Design review of the part built by this model. Coordinates are the model's own, in mm. A direction names the side the tool comes from. Coordinates: 2 decimals unless noted, no trailing zeros. Write each loop counter-clockwise with the first axis right and the second up, starting at its lowest first coordinate (ties: lowest second). Pieces come first, ordered by that corner, then holes. Notation, with made-up numbers: (22.5, -26.5) - (71.5, -26.5) arc R25 cw to (71.5, 1.5) - close; hole circle Ø6 at (40, 72). An arc over 180 degrees is marked (long way). Answer as CSV lines item,"result". Start each with the question number.
Q1. Machinability: for faces 1 (the face through (164.745, 9.658, -105.377)), 2 (the face through (223.617, 25.489, -167.34)), which of the approach directions +Z, -Z, +X, -X, +Y, -Y give a long, thin tool a straight path to every point of the face, cutting with its end or side? Answer none if there is none.
Q2. We need section C-C (y = 7.5). State how many separate pieces and enclosed holes the cut face has, plus the area to 3 significant figures.
Q3. We need section B-B (x = 136.5). Write out the cut boundary in (y, z).
Q4. For line 1 along Z through (x, y) = (47.5, 25.5); line 2 along Z through (x, y) = (46.5, 1.5); line 3 along Z through (x, y) = (91.5, 2), list the stretches that pass through material, from the lowest coordinate up. Write a range as [from, to].
Q5. We need section A-A (z = -25). Write out the cut boundary in (x, y), plus the area to 3 significant figures.
Q6. Mouldability with a two-part tool opening along Z and no side actions: class faces 3 (the face through (105.114, 9.658, -221.512)), 4 (the face through (131.43, 16.61, -271.15)), 5 (the face through (217.3, 9.658, -102.164)), 6 (the face through (269.77, 16.88, 3.14)) as pulls with the +Z half, pulls with the -Z half, needs draft (parallel to the pull), parting line crosses it, or undercut.
Q7. Clearance check with flat-ended pins moving along their axes: pin 1 (10 mm diameter, centred on y = 8, z = -64.5, fed in from -X); pin 2 (13.5 mm diameter, centred on x = 104.98, z = -48.24, fed in from +Y); pin 3 (1 mm diameter, centred on y = 4.5, z = -195, fed in from +X). State where each tip first meets the part, or that it passes through.
from build123d import *

# Parameters (mm, degrees)
SKETCH1_W           = 266.7
SKETCH1_H           = 266.7
BOSS_EXTRUDE1_DEPTH = 31.75
BOSS_EXTRUDE1_DRAFT = -15
SKETCH3_R           = 3.048
CUT_EXTRUDE1_DEPTH  = 31.75
SKETCH4_R           = 7.62
CUT_EXTRUDE2_DEPTH  = 12.7
FILLET1_R           = 5.08
FILLET2_R           = 2.54


with BuildPart() as part:
    # Sketch1 → Boss-Extrude1 (with draft: the straight prism first)
    with BuildSketch(Plane(origin=(0, 0, 0), x_dir=(1, 0, 0), z_dir=(0, 1, 0))):
        with Locations((133.35, 133.35)):
            Rectangle(SKETCH1_W, SKETCH1_H)
    extrude(amount=BOSS_EXTRUDE1_DEPTH)
    # Boss-Extrude1: the draft: its side faces are tilted about the plane it starts from
    boss_extrude1_sides = [part.faces().sort_by_distance(p)[0] for p in [
        (133.35, 15.875, 0),
        (266.7, 15.875, -133.35),
        (133.35, 15.875, -266.7),
        (0, 15.875, -133.35),
    ]]
    draft(boss_extrude1_sides, Plane(origin=(0, 0, 0), x_dir=(1, 0, 0), z_dir=(0, 1, 0)), BOSS_EXTRUDE1_DRAFT)

    # Sketch3 → Cut-Extrude1 (cut)
    with BuildSketch(Plane(origin=(0, 31.75, 0), x_dir=(1, 0, 0), z_dir=(0, 1, 0))):
        with Locations(Location((48.23621314, 48.23621314, 0), (0, 0, 270))):
            Circle(SKETCH3_R)
        with Locations(Location((104.97981314, 48.23621314, 0), (0, 0, 270))):
            Circle(SKETCH3_R)
        with Locations(Location((161.72341314, 48.23621314, 0), (0, 0, 270))):
            Circle(SKETCH3_R)
        with Locations(Location((218.46701314, 48.23621314, 0), (0, 0, 270))):
            Circle(SKETCH3_R)
        with Locations(Location((104.97981314, 104.97981314, 0), (0, 0, 270))):
            Circle(SKETCH3_R)
        with Locations(Location((161.72341314, 104.97981314, 0), (0, 0, 270))):
            Circle(SKETCH3_R)
        with Locations(Location((218.46701314, 104.97981314, 0), (0, 0, 270))):
            Circle(SKETCH3_R)
        with Locations(Location((104.97981314, 161.72341314, 0), (0, 0, 270))):
            Circle(SKETCH3_R)
        with Locations(Location((161.72341314, 161.72341314, 0), (0, 0, 270))):
            Circle(SKETCH3_R)
        with Locations(Location((218.46701314, 161.72341314, 0), (0, 0, 270))):
            Circle(SKETCH3_R)
        with Locations(Location((104.97981314, 218.46701314, 0), (0, 0, 270))):
            Circle(SKETCH3_R)
        with Locations(Location((161.72341314, 218.46701314, 0), (0, 0, 270))):
            Circle(SKETCH3_R)
        with Locations(Location((218.46701314, 218.46701314, 0), (0, 0, 270))):
            Circle(SKETCH3_R)
        with Locations(Location((48.23621314, 104.97981314, 0), (0, 0, 270))):
            Circle(SKETCH3_R)
        with Locations(Location((48.23621314, 161.72341314, 0), (0, 0, 270))):
            Circle(SKETCH3_R)
        with Locations(Location((48.23621314, 218.46701314, 0), (0, 0, 270))):
            Circle(SKETCH3_R)
    extrude(amount=-CUT_EXTRUDE1_DEPTH, mode=Mode.SUBTRACT)

    # Sketch4 → Cut-Extrude2 (cut)
    with BuildSketch(Plane(origin=(0, 31.75, 0), x_dir=(1, 0, 0), z_dir=(0, 1, 0))):
        with Locations(Location((218.46701314, 48.23621314, 0), (0, 0, 270))):
            Circle(SKETCH4_R)
        with Locations(Location((161.72341314, 48.23621314, 0), (0, 0, 270))):
            Circle(SKETCH4_R)
        with Locations(Location((104.97981314, 48.23621314, 0), (0, 0, 270))):
            Circle(SKETCH4_R)
        with Locations(Location((48.23621314, 48.23621314, 0), (0, 0, 270))):
            Circle(SKETCH4_R)
        with Locations(Location((161.72341314, 104.97981314, 0), (0, 0, 270))):
            Circle(SKETCH4_R)
        with Locations(Location((104.97981314, 104.97981314, 0), (0, 0, 270))):
            Circle(SKETCH4_R)
        with Locations(Location((48.23621314, 104.97981314, 0), (0, 0, 270))):
            Circle(SKETCH4_R)
        with Locations(Location((161.72341314, 161.72341314, 0), (0, 0, 270))):
            Circle(SKETCH4_R)
        with Locations(Location((104.97981314, 161.72341314, 0), (0, 0, 270))):
            Circle(SKETCH4_R)
        with Locations(Location((48.23621314, 161.72341314, 0), (0, 0, 270))):
            Circle(SKETCH4_R)
        with Locations(Location((161.72341314, 218.46701314, 0), (0, 0, 270))):
            Circle(SKETCH4_R)
        with Locations(Location((104.97981314, 218.46701314, 0), (0, 0, 270))):
            Circle(SKETCH4_R)
        with Locations(Location((48.23621314, 218.46701314, 0), (0, 0, 270))):
            Circle(SKETCH4_R)
        with Locations(Location((218.46701314, 104.97981314, 0), (0, 0, 270))):
            Circle(SKETCH4_R)
        with Locations(Location((218.46701314, 161.72341314, 0), (0, 0, 270))):
            Circle(SKETCH4_R)
        with Locations(Location((218.46701314, 218.46701314, 0), (0, 0, 270))):
            Circle(SKETCH4_R)
    extrude(amount=-CUT_EXTRUDE2_DEPTH, mode=Mode.SUBTRACT)

    # Fillet1
    fillet1_edges = [part.edges().sort_by_distance(p)[0] for p in [
        (-4.25369343, 15.875, -270.95369343),
        (270.95369343, 15.875, -270.95369343),
        (270.95369343, 15.875, 4.25369343),
        (-4.25369343, 15.875, 4.25369343),
    ]]
    fillet(fillet1_edges, radius=FILLET1_R)

    # Fillet2
    fillet2_edges = [part.edges().sort_by_distance(p)[0] for p in [
        (0, 0, -133.35),
        (133.35, 0, -266.7),
        (266.7, 0, -133.35),
        (133.35, 0, 0),
        (1.417846965, 0, -1.417846965),
        (265.282153035, 0, -1.417846965),
        (265.282153035, 0, -265.282153035),
        (1.417846965, 0, -265.282153035),
    ]]
    fillet(fillet2_edges, radius=FILLET2_R)


solid = part.part
Results list:
1,face 1,"+Y, -Y"
1,face 2,"+Y"
2,separate pieces,"1"
2,enclosed holes,"16"
2,area,"72,800 mm2"
3,outline,"(0, -264.75) arc R2.54 ccw to (1.88, -267.2) - (31.75, -275.21) - (31.75, 8.51) - (1.88, 0.5) arc R2.54 ccw to (0, -1.95) - close"
4,line 1,"z = [-273.53, -226.05], [-210.88, -169.31], [-154.14, -112.56], [-97.4, -55.82], [-40.65, 6.83]"
4,line 2,"z = [-267.07, -220.97], [-215.96, -164.23], [-159.22, -107.48], [-102.47, -50.74], [-45.73, 0.37]"
4,line 3,"z = [-267.24, 0.54]"
5,outline,"(-8.51, 31.75) - (-0.5, 1.88) arc R2.54 ccw to (1.95, 0) - (264.75, 0) arc R2.54 ccw to (267.2, 1.88) - (275.21, 31.75) - close"
5,area,"8,740 mm2"
6,face 3,"undercut"
6,face 4,"pulls with the -Z half"
6,face 5,"undercut"
6,face 6,"pulls with the +Z half"
7,pin 1,"stops at x = -3.48"
7,pin 2,"stops at y = 19.05"
7,pin 3,"stops at x = 268.04"
